Check sheet for the modelled part. Datum: model origin and axes. Units: mm. Give positions to 0.01 mm unless a question says otherwise; leave off trailing zeros. Order: outer loops, then holes, each group sorted by start corner. A loop starts at its lowest first (then second) coordinate and runs counter-clockwise, first axis right, second up.
Autodesk Inventor part; units mm, degrees
ref_plane "YZ Plane" through (0, 0, 0) normal (1, 0, 0) x (0, 1, 0)
ref_plane "XZ Plane" through (0, 0, 0) normal (0, 1, 0) x (-1, 0, 0)
ref_plane "XY Plane" through (0, 0, 0) normal (0, 0, 1) x (1, 0, 0)
sketch "スケッチ1" plane through (0, 0, 0) normal (0, 1, 0) x (-1, 0, 0)
  line L0 (0, 0) -> (5.08, 0)
  line L1 (5.08, 0) -> (2.54, 0)
  line L2 (2.54, 0) -> (0, 0)
  line L3 (0, 0) -> (-2.54, 0)
  line L4 (-2.54, 0) -> (-5.08, 0)
  circle A0 centre (-2.54, 0) radius 0.4
  circle A1 centre (0, 0) radius 0.4
  circle A2 centre (2.54, 0) radius 0.4
  circle A3 centre (5.08, 0) radius 0.4
  line L5 (0, 0) -> (1.27, 0)
  line L6 (-3.73, -1) -> (6.27, -1)
  line L7 (6.27, -1) -> (6.27, 1)
  line L8 (6.27, 1) -> (-3.73, 1)
  line L9 (-3.73, 1) -> (-3.73, -1)
  line L10 (-3.73, -1) -> (6.27, 1) construction
  line L11 (6.27, -1) -> (-3.73, 1) construction
  line L12 (4.68, -0.4) -> (5.48, -0.4)
  line L13 (5.48, -0.4) -> (5.48, 0.4)
  line L14 (5.48, 0.4) -> (4.68, 0.4)
  line L15 (4.68, 0.4) -> (4.68, -0.4)
  line L16 (4.68, -0.4) -> (5.48, 0.4) construction
  line L17 (5.48, -0.4) -> (4.68, 0.4) construction
  line L18 (2.14, -0.4) -> (2.94, -0.4)
  line L19 (2.94, -0.4) -> (2.94, 0.4)
  line L20 (2.94, 0.4) -> (2.14, 0.4)
  line L21 (2.14, 0.4) -> (2.14, -0.4)
  line L22 (2.14, -0.4) -> (2.94, 0.4) construction
  line L23 (2.94, -0.4) -> (2.14, 0.4) construction
  line L24 (-0.4, -0.4) -> (0.4, -0.4)
  line L25 (0.4, -0.4) -> (0.4, 0.4)
  line L26 (0.4, 0.4) -> (-0.4, 0.4)
  line L27 (-0.4, 0.4) -> (-0.4, -0.4)
  line L28 (-0.4, -0.4) -> (0.4, 0.4) construction
  line L29 (0.4, -0.4) -> (-0.4, 0.4) construction
  line L30 (-2.94, -0.4) -> (-2.14, -0.4)
  line L31 (-2.14, -0.4) -> (-2.14, 0.4)
  line L32 (-2.14, 0.4) -> (-2.94, 0.4)
  line L33 (-2.94, 0.4) -> (-2.94, -0.4)
  line L34 (-2.94, -0.4) -> (-2.14, 0.4) construction
  line L35 (-2.14, -0.4) -> (-2.94, 0.4) construction
  dimension "d0" = 5.08
  dimension "d1" = 2.54
  dimension "d2" = 2.54
  dimension "d3" = 2.54
  dimension "d4" = 0.8
  dimension "d5" = 0.8
  dimension "d6" = 0.8
  dimension "d7" = 0.8
  dimension "d8" = 1.27
  dimension "d9" = 10
  dimension "d10" = 2
extrude "押し出し1" add sketch "スケッチ1" along normal blind 4.8
properties part number "ikafly8_2.54"
(1) Cross-section at A-A on x = -2.5. Enter the section's corners in (y, z).
Response values:
outline: (0, -1) - (4.8, -1) - (4.8, -0.4) - (0, -0.4) - close; (0, 0.4) - (4.8, 0.4) - (4.8, 1) - (0, 1) - close
(2) Cross-section at C-C on y = 3.45. Enter the section's corners in (x, z).
Response values:
outline: (-6.27, -1) - (3.73, -1) - (3.73, 1) - (-6.27, 1) - close; hole (-5.48, -0.4) - (-4.68, -0.4) - (-4.68, 0.4) - (-5.48, 0.4) - close; hole (-2.94, -0.4) - (-2.14, -0.4) - (-2.14, 0.4) - (-2.94, 0.4) - close; hole (-0.4, -0.4) - (0.4, -0.4) - (0.4, 0.4) - (-0.4, 0.4) - close; hole (2.14, -0.4) - (2.94, -0.4) - (2.94, 0.4) - (2.14, 0.4) - close
(3) Material ranges on L1, parallel to X at y = 1.3, z = 0.1; L2, parallel to Z at x = -2.75, y = 2.35, recorded low to high.
Response values:
L1: x = -6.27 to -5.48, -4.68 to -2.94, -2.14 to -0.4, 0.4 to 2.14, 2.94 to 3.73
L2: z = -1 to -0.4, 0.4 to 1
(4) Release check for a two-part mould opening along Z. For faces 1 (the face through (-1, 2, 1)), 2 (the face through (-6.27, 2, 0)), 3 (the face through (-5, 2, -0.4)), 4 (the face through (-5, 2, 0.4)) record: released by +Z, released by -Z, zero draft, split by the parting line, or undercut.
Response values:
face 1: released by +Z
face 2: zero draft
face 3: undercut
face 4: undercut
(5) Cross-section at B-B on z = 0.25. Enter the section's corners in (x, y), then the cut area to 3 significant figures.
Response values:
outline: (-6.27, 0) - (-5.48, 0) - (-5.48, 4.8) - (-6.27, 4.8) - close; (-4.68, 0) - (-2.94, 0) - (-2.94, 4.8) - (-4.68, 4.8) - close; (-2.14, 0) - (-0.4, 0) - (-0.4, 4.8) - (-2.14, 4.8) - close; (0.4, 0) - (2.14, 0) - (2.14, 4.8) - (0.4, 4.8) - close; (2.94, 0) - (3.73, 0) - (3.73, 4.8) - (2.94, 4.8) - close
area: 32.6 mm2
